Check sheet for the modelled part. Datum: model origin and axes. Units: mm. A direction names the side the tool comes from. Give positions to 0.01 mm unless a question says otherwise; leave off trailing zeros. Loops run counter-clockwise (first coordinate to the right, second up) from the corner with the lowest first, then second, coordinate; pieces in that order, holes last. Notation, with made-up numbers: M -18.5,-38.5 L 7.5,-38.5 A31 ccw 7.5,0.5 Z; hole C 65,87.5 d5. An arc over 180 degrees is marked long. Put each result on its own line as item: value. Start each with the question number.
```python
from build123d import *

# Parameters (mm, degrees)
F0_R      = 17.78
F0_R_2    = 15.24
F1_DEPTH  = 17.78
F2_R      = 17.78
F3_DEPTH  = 5.08
F4_R      = 1.524
F5_DEPTH  = 25.4
F6_R      = 27.94
F6_R_2    = 2.159
F6_R_3    = 9.525
F7_DEPTH  = 5.08
F8_SIZE   = 5.07999
F10_DEPTH = 3.81


# Not quite as in the source:
# - a fillet or chamfer is up to 0.001 mm smaller than in the source, because OpenCascade refuses the exact size


with BuildPart() as f1:
    # F0 (on Right) → F1 (new body)
    with BuildSketch(Plane.YZ):
        Circle(F0_R)
        Circle(F0_R_2, mode=Mode.SUBTRACT)
    extrude(amount=F1_DEPTH)

    # F2 (on face) → F3 (join)
    with BuildSketch(Plane.YZ.offset(17.78)):
        Circle(F2_R)
    extrude(amount=F3_DEPTH)

    # F4 (on face) → F5 (cut)
    with BuildSketch(Plane.YZ.offset(22.86)):
        Circle(F4_R)
    extrude(amount=-F5_DEPTH, mode=Mode.SUBTRACT)

    # F6 (on face) → F7 (join)
    with BuildSketch(Plane.YZ.offset(22.86)):
        Circle(F6_R)
        with Locations((0, -23.8125)):
            Circle(F6_R_2, mode=Mode.SUBTRACT)
        with Locations((-20.6222299276, -11.90625)):
            Circle(F6_R_2, mode=Mode.SUBTRACT)
        Circle(F6_R_3, mode=Mode.SUBTRACT)
        with Locations((20.6222299276, -11.90625)):
            Circle(F6_R_2, mode=Mode.SUBTRACT)
        with Locations((-20.6222299276, 11.90625)):
            Circle(F6_R_2, mode=Mode.SUBTRACT)
        with Locations((0, 23.8125)):
            Circle(F6_R_2, mode=Mode.SUBTRACT)
        with Locations((20.6222299276, 11.90625)):
            Circle(F6_R_2, mode=Mode.SUBTRACT)
    extrude(amount=F7_DEPTH)

    # F8 (size 5.08 in the source; OpenCascade refuses exactly that, so slightly less here)
    f8_edges = [f1.edges().sort_by_distance(p)[0] for p in [
        (27.94, -9.525, 0),
    ]]
    chamfer(f8_edges, length=F8_SIZE)

    # F9 (on face) → F10 (cut)
    with BuildSketch(Plane(origin=(17.78, 0, 0), x_dir=(0, -1, 0), z_dir=(-1, 0, 0))):
        with BuildLine():
            ThreePointArc((3.3655, 2.413), (0, 4.437080139), (-3.3655, 2.413))
            Line((-3.3655, 2.413), (-3.3655, -2.413))
            ThreePointArc((-3.3655, -2.413), (0, -4.437080139), (3.3655, -2.413))
            Line((3.3655, -2.413), (3.3655, 2.413))
        make_face()
    extrude(amount=-F10_DEPTH, mode=Mode.SUBTRACT)


solid = f1.part
```
Q1. Section check D-D, the plane x = 12.5. Record the cut outline in (y, z), then the cut area to 3 significant figures.
Q2. Mould release check, pull along Y, two halves, no side actions. Record for faces 4 (the face through (0, -8, 13.3)), 5 (the face through (25.36, -3.64, 27.7)), 6 (the face through (21.59, 2, 0)): pulls with the +Y half, pulls with the -Y half, needs draft (parallel to the pull), parting line crosses it, or undercut.
Q3. Access from +Z, -Z, +X, -X, +Y, -Y to the whole of each face (thin tool, end or side, straight path). Record for faces 1 (the face through (22.23, -0.2, 1.51)), 2 (the face through (20, 3.366, 0)), 3 (the face through (22.86, 2, 0)).
Q4. Section check C-C, the plane x = 19.75. Record the cut outline in (y, z), then the cut area to 3 significant figures.
Q5. Depth check by flat-ended pin: P1, Ø3, axis at x = 19.5, z = 1, coming from the -Y side; P2, Ø3, axis at x = 19, z = 0.5, coming from the +Y side; P3, Ø5, axis at y = 0, z = 23.81, coming from the -X side. Enter the tip coordinate at first touch or a pass-through.
Q6. Section check A-A, the plane y = 0. Give the number of separate pieces and of enclosed holes in the cut face, then the cut area to 3 significant figures.
Q7. Thickness scan on line 1 along Z through (x, y) = (22.4, 0); line 2 along Z through (x, y) = (13.5, 0); line 3 along Z through (x, y) = (26.75, -20.5). Record the ranges inside material, lowest first. Write a range as [from, to].
Found:
1. outline: C 0,0 d35.56; hole C 0,0 d30.48
1. area: 263 mm^2
2. face 4: needs draft
2. face 5: parting line crosses it
2. face 6: undercut
3. face 1: +X, -X
3. face 2: -X
3. face 3: +X
4. outline: C 0,0 d35.56; hole M -3.37,-2.41 A3.81 ccw 3.37,-2.41 L 3.37,2.41 A3.81 ccw -3.37,2.41 Z
4. area: 941 mm^2
5. P1: stops at y = -17.78
5. P2: stops at y = 17.78
5. P3: stops at x = 22.86
6. separate pieces: 4
6. enclosed holes: 0
6. area: 351 mm^2
7. line 1: z = [-17.78, -1.52], [1.52, 17.78]
7. line 2: z = [-17.78, -15.24], [15.24, 17.78]
7. line 3: z = [-18.98, -14.06], [-9.75, 9.75], [14.06, 18.98]
